Verification items for the finished model (mm, model axes). A direction names the side the tool comes from. Give positions to 0.01 mm unless a question says otherwise; leave off trailing zeros. Loops run counter-clockwise (first coordinate to the right, second up) from the corner with the lowest first, then second, coordinate; pieces in that order, holes last. Notation, with made-up numbers: (15.25, 75) - (39.25, 75) arc R20 ccw to (39.25, 114) - close; hole circle Ø2 at (22, 9). An arc over 180 degrees is marked (long way). Use one line per item in the form item = value.
```python
from build123d import *

# Parameters (mm, degrees)
SKETCH_1_R      = 3
SKETCH_1_R_2    = 1.6
EXTRUDE_1_DEPTH = 5


with BuildPart() as part:
    # ｽｹｯﾁ1 → ﾎﾞｽ - 押し出し1 (new body)
    with BuildSketch(Plane.XY):
        Polygon((0, -6), (50, -6), (50, 6), (47.5, 6), (47.5, -4), (44.5, -4), (44.5, 6), (-10, 6), (-10, -6), align=None)
        Circle(SKETCH_1_R, mode=Mode.SUBTRACT)
        with Locations((5.629165125, 3.25)):
            Circle(SKETCH_1_R_2, mode=Mode.SUBTRACT)
        with Locations((-5.629165125, -3.25)):
            Circle(SKETCH_1_R_2, mode=Mode.SUBTRACT)
    extrude(amount=EXTRUDE_1_DEPTH)


solid = part.part
```
1. Draft check along X on faces 1 (the cylindrical face through (-3, 0, 2)), 2 (the flat face through (20, 0, 0)), 3 (the flat face through (50, 0, 2)). Enter one of: released by +X, released by -X, zero draft, split by the parting line, or undercut.
Result set:
face_1 = undercut
face_2 = zero draft
face_3 = released by +X
2. Section check A-A, the plane y = 0. Record the cut outline in (x, z).
Result set:
outline = (-10, 0) - (-3, 0) - (-3, 5) - (-10, 5) - close; (3, 0) - (44.5, 0) - (44.5, 5) - (3, 5) - close; (47.5, 0) - (50, 0) - (50, 5) - (47.5, 5) - close
3. Scan lines: probe 1 along Y at (x, z) = (0, 1.4); probe 2 along X at (y, z) = (-1.25, 2.5); probe 3 along X at (y, z) = (-1.5, 3.3). Record each from-to range of solid material in increasing order.
Result set:
probe_1 = -6 to -3, 3 to 6
probe_2 = -10 to -2.73, 2.73 to 44.5, 47.5 to 50
probe_3 = -10 to -2.6, 2.6 to 44.5, 47.5 to 50
4. Section check D-D, the plane y = -2.5. Record the cut outline in (x, z).
Result set:
outline = (-10, 0) - (-7.04, 0) - (-7.04, 5) - (-10, 5) - close; (-4.22, 0) - (-1.66, 0) - (-1.66, 5) - (-4.22, 5) - close; (1.66, 0) - (44.5, 0) - (44.5, 5) - (1.66, 5) - close; (47.5, 0) - (50, 0) - (50, 5) - (47.5, 5) - close
5. Tool access check on faces 4 (the flat face through (44.5, 1, 2)), 5 (the flat face through (18, 6, 2)). Record the directions out of +Z, -Z, +X, -X, +Y, -Y that give a thin tool (end or side, any length) a straight path to the whole face; none if there is none.
Result set:
face_4 = +Z, -Z, +Y
face_5 = +Z, -Z, +X, -X, +Y
6. Depth check by flat-ended pin: pin 1 Ø0.9 at (x, z) = (46.5, 2.5) entering from +Y. Enter the tip coordinate at first touch or a pass-through.
Result set:
pin_1 = -4
7. Section check B-B, the plane x = 0. Record the cut outline in (y, z), then the cut area to 3 significant figures.
Result set:
outline = (-6, 0) - (-3, 0) - (-3, 5) - (-6, 5) - close; (3, 0) - (6, 0) - (6, 5) - (3, 5) - close
area = 30.0 mm²
8. Section check C-C, the plane z = 1.2. Record the cut outline in (x, y).
Result set:
outline = (-10, -6) - (50, -6) - (50, 6) - (47.5, 6) - (47.5, -4) - (44.5, -4) - (44.5, 6) - (-10, 6) - close; hole circle Ø3.2 at (-5.63, -3.25); hole circle Ø6 at (0, 0); hole circle Ø3.2 at (5.63, 3.25)
